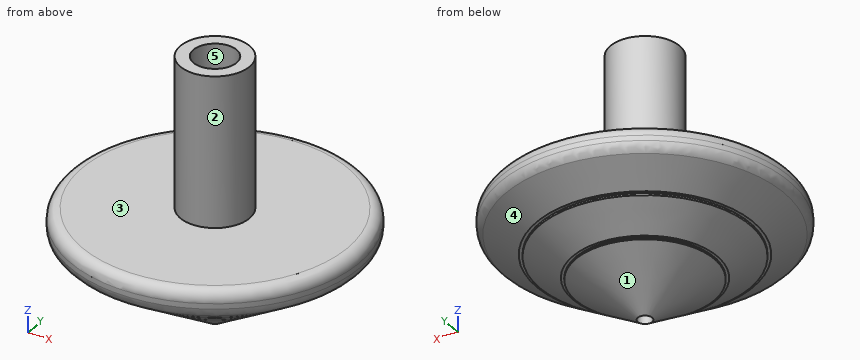
```python
from build123d import *

# Parameters (mm, degrees)
F2_R      = 2.54
F3_R      = 1.5875
F4_DEPTH  = 8.5725
F5_R      = 4.7625
F6_DEPTH  = 42.545
F7_R      = 17.565268
F7_R_2    = 15.226775
F8_DEPTH  = 10.16
F9_R      = 24.251391
F9_R_2    = 23.10866
F10_DEPTH = 15.24


with BuildPart() as f1:
    # F0 (on Front) → F1 (revolve)
    with BuildSketch(Plane.XZ):
        Polygon((0, 58.42), (0, 0), (31.75, 20.32), (31.75, 25.4), (7.62, 25.4), (7.62, 58.42), align=None)
    revolve(axis=Axis((0, 0, 29.21), (0, 0, -1)))

    # F2
    f2_edges = [f1.edges().sort_by_distance(p)[0] for p in [
        (-31.75, 0, 20.32),
        (-31.75, 0, 25.4),
        (31.75, 0, 22.86),
    ]]
    fillet(f2_edges, radius=F2_R)

    # F3 (on Top) → F4 (cut)
    with BuildSketch(Plane.XY):
        Circle(F3_R)
    extrude(amount=F4_DEPTH, mode=Mode.SUBTRACT)

    # F5 (on face) → F6 (cut)
    with BuildSketch(Plane.XY.offset(58.42)):
        Circle(F5_R)
    extrude(amount=-F6_DEPTH, mode=Mode.SUBTRACT)

    # F7 (on Top) → F8 (cut)
    with BuildSketch(Plane.XY):
        Circle(F7_R)
        Circle(F7_R_2, mode=Mode.SUBTRACT)
    extrude(amount=F8_DEPTH, mode=Mode.SUBTRACT)

    # F9 (on Top) → F10 (cut)
    with BuildSketch(Plane.XY):
        Circle(F9_R)
        Circle(F9_R_2, mode=Mode.SUBTRACT)
    extrude(amount=F10_DEPTH, mode=Mode.SUBTRACT)


solid = f1.part
```
Verification items for the finished model (mm, model axes). Face numbers are marked on the shaded views. A direction names the side the tool comes from. Coordinates: 2 decimals unless noted, no trailing zeros. Order: outer loops, then holes, each group sorted by start corner. A loop starts at its lowest first (then second) coordinate and runs counter-clockwise, first axis right, second up. Notation, with made-up numbers: (75.25, 9) -> (120.25, 9) arc R20 cw to (120.25, 24) -> close; hole circle Ø10 at (-0.75, 62). An arc over 180 degrees is marked (long way). Put each result on its own line as item: value. Start each with the question number.
1) Release check for a two-part mould opening along X. For the marked faces 3, 4 and 5 record: pulls with the +X half, pulls with the -X half, needs draft (parallel to the pull), parting line crosses it, or undercut.
2) Material ranges on L1, parallel to Y at x = 0, z = 27; L2, parallel to X at y = 4, z = 20; L3, parallel to Y at x = 0, z = 4.5, recorded low to high.
3) Cross-section at A-A (z = 32). Enter the section's corners in (x, y) (1 decimal), plus the area to 3 significant figures.
4) Cross-section at B-B (z = 5). Enter the section's corners in (x, y) (1 decimal).
5) Tool access check on the marked faces 1 and 2. Record the directions out of +Z, -Z, +X, -X, +Y, -Y that give a thin tool (end or side, any length) a straight path to the whole face; none if there is none.
6) Go/stop test with flat-tipped pins: pin 1 (2 mm diameter, centred on y = -11.5, z = 27, fed in from -X); pin 2 (2 mm diameter, centred on x = -11.5, y = -0.5, fed in from -Z); pin 3 (5 mm diameter, centred on x = -17.5, y = 6.5, fed in from +Z); pin 4 (6 mm diameter, centred on x = 17, y = -24.5, fed in from -Z) (3 decimals). Record where each tip stops, or that it passes through.
Geometry check:
1. face 3: needs draft
1. face 4: parting line crosses it
1. face 5: undercut
2. L1: y = -7.62 to -4.76, 4.76 to 7.62
2. L2: x = -30.83 to -2.58, 2.58 to 30.83
2. L3: y = -7.03 to -1.59, 1.59 to 7.03
3. outline: circle Ø15.2 at (0, 0); hole circle Ø9.5 at (0, 0)
3. area: 111 mm^2
4. outline: circle Ø15.6 at (0, 0); hole circle Ø3.2 at (0, 0)
5. face 1: -Z
5. face 2: +Z
6. pin 1: passes through
6. pin 2: stops at z = 6.73
6. pin 3: stops at z = 25.4
6. pin 4: stops at z = 17.165
